Work out the finished part from the listing and answer in its coordinate system (mm). Round coordinates to 2 decimals unless told otherwise and drop trailing zeros. Return JSON: item names as keys, results as strings.
from build123d import *

# Parameters (mm, degrees)
F0_R     = 213.7585
F0_R_2   = 194.315
F1_DEPTH = 6
F2_R     = 3
F3_DEPTH = 6.001


with BuildPart() as f1:
    # F0 (on Top) → F1 (new body)
    with BuildSketch(Plane.XY):
        Circle(F0_R)
        Circle(F0_R_2, mode=Mode.SUBTRACT)
    extrude(amount=F1_DEPTH)

    # F2 (on face) → F3 (cut, through all)
    with BuildSketch(Plane.XY.offset(6)):
        with Locations((0, 204.037)):
            Circle(F2_R)
        with Locations((-15.247704, 203.466471)):
            Circle(F2_R)
        with Locations((-30.410137, 201.758075)):
            Circle(F2_R)
        with Locations((-45.402504, 198.921366)):
            Circle(F2_R)
        with Locations((-60.140962, 194.972209)):
            Circle(F2_R)
        with Locations((-74.543087, 189.932687)):
            Circle(F2_R)
        with Locations((-88.528336, 183.830985)):
            Circle(F2_R)
        with Locations((-102.0185, 176.701225)):
            Circle(F2_R)
        with Locations((-114.938135, 168.583281)):
            Circle(F2_R)
        with Locations((-127.214989, 159.52255)):
            Circle(F2_R)
        with Locations((-138.780405, 149.569705)):
            Circle(F2_R)
        with Locations((-149.569705, 138.780405)):
            Circle(F2_R)
        with Locations((-159.52255, 127.214989)):
            Circle(F2_R)
        with Locations((-168.583281, 114.938135)):
            Circle(F2_R)
        with Locations((-176.701225, 102.0185)):
            Circle(F2_R)
        with Locations((-183.830985, 88.528336)):
            Circle(F2_R)
        with Locations((-189.932687, 74.543087)):
            Circle(F2_R)
        with Locations((-194.972209, 60.140962)):
            Circle(F2_R)
        with Locations((-198.921366, 45.402504)):
            Circle(F2_R)
        with Locations((-201.758075, 30.410137)):
            Circle(F2_R)
        with Locations((-203.466471, 15.247704)):
            Circle(F2_R)
        with Locations((-204.037, 0)):
            Circle(F2_R)
        with Locations((-203.466471, -15.247704)):
            Circle(F2_R)
        with Locations((-201.758075, -30.410137)):
            Circle(F2_R)
        with Locations((-198.921366, -45.402504)):
            Circle(F2_R)
        with Locations((-194.972209, -60.140962)):
            Circle(F2_R)
        with Locations((-189.932687, -74.543087)):
            Circle(F2_R)
        with Locations((-183.830985, -88.528336)):
            Circle(F2_R)
        with Locations((-176.701225, -102.0185)):
            Circle(F2_R)
        with Locations((-168.583281, -114.938135)):
            Circle(F2_R)
        with Locations((-159.52255, -127.214989)):
            Circle(F2_R)
        with Locations((-149.569705, -138.780405)):
            Circle(F2_R)
        with Locations((-138.780405, -149.569705)):
            Circle(F2_R)
        with Locations((-127.214989, -159.52255)):
            Circle(F2_R)
        with Locations((-114.938135, -168.583281)):
            Circle(F2_R)
        with Locations((-102.0185, -176.701225)):
            Circle(F2_R)
        with Locations((-88.528336, -183.830985)):
            Circle(F2_R)
        with Locations((-74.543087, -189.932687)):
            Circle(F2_R)
        with Locations((-60.140962, -194.972209)):
            Circle(F2_R)
        with Locations((-45.402504, -198.921366)):
            Circle(F2_R)
        with Locations((-30.410137, -201.758075)):
            Circle(F2_R)
        with Locations((-15.247704, -203.466471)):
            Circle(F2_R)
        with Locations((0, -204.037)):
            Circle(F2_R)
        with Locations((15.247704, -203.466471)):
            Circle(F2_R)
        with Locations((30.410137, -201.758075)):
            Circle(F2_R)
        with Locations((45.402504, -198.921366)):
            Circle(F2_R)
        with Locations((60.140962, -194.972209)):
            Circle(F2_R)
        with Locations((74.543087, -189.932687)):
            Circle(F2_R)
        with Locations((88.528336, -183.830985)):
            Circle(F2_R)
        with Locations((102.0185, -176.701225)):
            Circle(F2_R)
        with Locations((114.938135, -168.583281)):
            Circle(F2_R)
        with Locations((127.214989, -159.52255)):
            Circle(F2_R)
        with Locations((138.780405, -149.569705)):
            Circle(F2_R)
        with Locations((149.569705, -138.780405)):
            Circle(F2_R)
        with Locations((159.52255, -127.214989)):
            Circle(F2_R)
        with Locations((168.583281, -114.938135)):
            Circle(F2_R)
        with Locations((176.701225, -102.0185)):
            Circle(F2_R)
        with Locations((183.830985, -88.528336)):
            Circle(F2_R)
        with Locations((189.932687, -74.543087)):
            Circle(F2_R)
        with Locations((194.972209, -60.140962)):
            Circle(F2_R)
        with Locations((198.921366, -45.402504)):
            Circle(F2_R)
        with Locations((201.758075, -30.410137)):
            Circle(F2_R)
        with Locations((203.466471, -15.247704)):
            Circle(F2_R)
        with Locations((204.037, 0)):
            Circle(F2_R)
        with Locations((203.466471, 15.247704)):
            Circle(F2_R)
        with Locations((201.758075, 30.410137)):
            Circle(F2_R)
        with Locations((198.921366, 45.402504)):
            Circle(F2_R)
        with Locations((194.972209, 60.140962)):
            Circle(F2_R)
        with Locations((189.932687, 74.543087)):
            Circle(F2_R)
        with Locations((183.830985, 88.528336)):
            Circle(F2_R)
        with Locations((176.701225, 102.0185)):
            Circle(F2_R)
        with Locations((168.583281, 114.938135)):
            Circle(F2_R)
        with Locations((159.52255, 127.214989)):
            Circle(F2_R)
        with Locations((149.569705, 138.780405)):
            Circle(F2_R)
        with Locations((138.780405, 149.569705)):
            Circle(F2_R)
        with Locations((127.214989, 159.52255)):
            Circle(F2_R)
        with Locations((114.938135, 168.583281)):
            Circle(F2_R)
        with Locations((102.0185, 176.701225)):
            Circle(F2_R)
        with Locations((88.528336, 183.830985)):
            Circle(F2_R)
        with Locations((74.543087, 189.932687)):
            Circle(F2_R)
        with Locations((60.140962, 194.972209)):
            Circle(F2_R)
        with Locations((45.402504, 198.921366)):
            Circle(F2_R)
        with Locations((30.410137, 201.758075)):
            Circle(F2_R)
        with BuildLine():
            ThreePointArc((15.018019, 200.475277), (17.286202, 201.265442), (18.247704, 203.466471))
            ThreePointArc((18.247704, 203.466471), (13.209207, 205.6675), (15.018019, 200.475277))
        make_face()
    extrude(amount=-F3_DEPTH, mode=Mode.SUBTRACT)


solid = f1.part
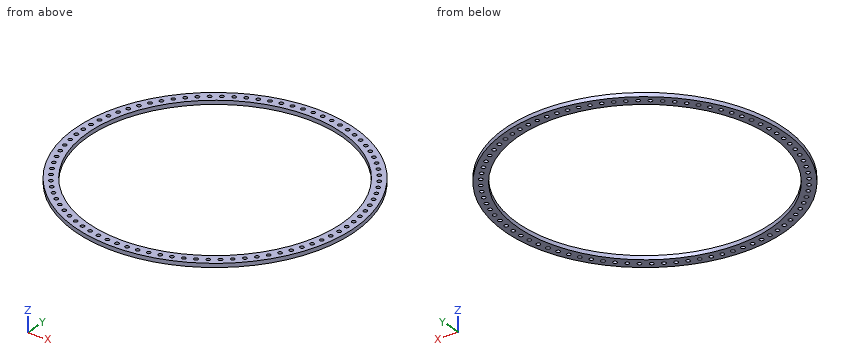
Item 1: Each of these flat-tipped pins is pushed along its axis until it touches: pin 1 (9.5 mm diameter, centred on x = 183.83, y = -88.53, fed in from +Z); pin 2 (1.5 mm diameter, centred on y = -61, z = 5, fed in from -X). Where does it stop, or does it pass through?
Output:
{"pin 1": "stops at z = 6", "pin 2": "stops at x = -205.09"}
Item 2: Consider line 1 along Y through (x, z) = (0, 3.2) (1 decimal); line 2 along X through (y, z) = (88, 3); line 3 along Y through (x, z) = (-115, 5.4). Determine where each line is inside the solid, lowest interval first. Write a range as [from, to].
Output:
{"line 1": "y = [-213.8, -207], [-201, -194.3], [194.3, 201], [207, 213.8]", "line 2": "x = [-194.8, -186.78], [-180.88, -173.25], [173.25, 180.88], [186.78, 194.8]", "line 3": "y = [-180.19, -171.58], [-165.58, -156.63], [156.63, 165.58], [171.58, 180.19]"}
Item 3: Find section A-A (z = 4.9). State how many separate pieces and enclosed holes the cut face has, plus the area to 3 significant figures.
Output:
{"separate pieces": "1", "enclosed holes": "85", "area": "22,600 mm^2"}
